Check sheet for the modelled part. Datum: model origin and axes. Units: mm. A direction names the side the tool comes from. Coordinates: 2 decimals unless noted, no trailing zeros. Loops run counter-clockwise (first coordinate to the right, second up) from the corner with the lowest first, then second, coordinate; pieces in that order, holes last. Notation, with made-up numbers: M 51,7.5 L 64,7.5 A17 cw 64,34.5 Z; hole C -11.5,-5 d9. An arc over 180 degrees is marked long. Return JSON: item names as keys, results as strings.
from build123d import *

# Parameters (mm, degrees)
SKETCH1_R           = 5.842
BOSS_EXTRUDE1_DEPTH = 1.397
SKETCH2_R           = 5.588
CUT_EXTRUDE1_DEPTH  = 0.381
SKETCH3_R           = 3.175
CUT_EXTRUDE2_DEPTH  = 9.324072561
SKETCH4_R           = 3.81
BOSS_EXTRUDE2_DEPTH = 0.381
CHAMFER1_SIZE       = 0.381
SKETCH5_R           = 3.175
CUT_EXTRUDE3_DEPTH  = 9.379113139


with BuildPart() as part:
    # Sketch1 → Boss-Extrude1 (new body)
    with BuildSketch(Plane(origin=(0, 0, 0), x_dir=(0, 0, -1), z_dir=(1, 0, 0))):
        Circle(SKETCH1_R)
    extrude(amount=BOSS_EXTRUDE1_DEPTH)

    # Sketch2 → Cut-Extrude1 (cut)
    with BuildSketch(Plane(origin=(1.397, 0, 0), x_dir=(0, 0, -1), z_dir=(1, 0, 0))):
        Circle(SKETCH2_R)
    extrude(amount=-CUT_EXTRUDE1_DEPTH, mode=Mode.SUBTRACT)

    # Sketch3 → Cut-Extrude2 (cut, through all)
    with BuildSketch(Plane(origin=(1.016, 0, 0), x_dir=(0, 0, -1), z_dir=(1, 0, 0))):
        Circle(SKETCH3_R)
    extrude(amount=-CUT_EXTRUDE2_DEPTH, mode=Mode.SUBTRACT)

    # Sketch4 → Boss-Extrude2 (add)
    with BuildSketch(Plane.ZY):
        with Locations(Location((0, 0, 0), (0, 0, 180))):
            Circle(SKETCH4_R)
    extrude(amount=BOSS_EXTRUDE2_DEPTH)

    # Chamfer1
    chamfer1_edges = [part.edges().sort_by_distance(p)[0] for p in [
        (0, 0, 3.81),
    ]]
    chamfer(chamfer1_edges, length=CHAMFER1_SIZE - 0.0001)  # a hair under: the kernel refuses the full size

    # Sketch5 → Cut-Extrude3 (cut, through all)
    with BuildSketch(Plane(origin=(0, 0, 0), x_dir=(0, 0, -1), z_dir=(1, 0, 0))):
        Circle(SKETCH5_R)
    extrude(amount=-CUT_EXTRUDE3_DEPTH, mode=Mode.SUBTRACT)


solid = part.part
1) Section check C-C on x = 0.2. Record the cut outline in (y, z) (3 decimals).
Answers:
{"outline": "C 0,0 d11.684; hole C 0,0 d6.35"}
2) Set-up check for faces 1 (the face through (1.016, -2.4, -2.4)), 2 (the face through (0, -4, -3)), 3 (the face through (0.33, -3.1, 0.69)): record each of +Z, -Z, +X, -X, +Y, -Y from which the full face is reachable in a straight line by a thin tool's end or side.
Answers:
{"face 1": "+X", "face 2": "-X", "face 3": "+X, -X"}
3) Draft check along Z on faces 4 (the face through (0.689, -5.703, 1.266)), 5 (the face through (-0.381, -3, 2)), 6 (the face through (1.209, -3.4, 4.434)). Enter one of: +Z half, -Z half, draft (parallel to the pull), parting line (faces both ways), or undercut.
Answers:
{"face 4": "parting line", "face 5": "draft", "face 6": "undercut"}
4) Section check D-D on y = -5. Record the cut outline in (x, z), then the cut area to 3 significant figures.
Answers:
{"outline": "M 0,-3.02 L 1.4,-3.02 L 1.4,-2.5 L 1.02,-2.5 L 1.02,2.5 L 1.4,2.5 L 1.4,3.02 L 0,3.02 Z", "area": "6.54 mm²"}
5) Go/stop test with a flat-tipped pin: pin 1 Ø3.5 at (y, z) = (-2, 1) entering from +X. Record where the tip stops, or that it passes through.
Answers:
{"pin 1": "x = 1.02"}
6) Scan lines: line 1 along Y through (x, z) = (0.65, 0) (3 decimals); line 2 along Y through (x, z) = (1.2, 0); line 3 along X through (y, z) = (-3.5, 3.5). Record each from-to range of solid material in increasing order. Write a range as [from, to].
Answers:
{"line 1": "[-5.842, -3.175], [3.175, 5.842]", "line 2": "[-5.84, -5.59], [5.59, 5.84]", "line 3": "[0, 1.02]"}
